Design review of the part built by this model. Coordinates are the model's own, in mm. Face numbers are marked on the shaded views. A direction names the side the tool comes from. Coordinates: 2 decimals unless noted, no trailing zeros. Loops run counter-clockwise (first coordinate to the right, second up) from the corner with the lowest first, then second, coordinate; pieces in that order, holes last. Notation, with made-up numbers: (-17.75, 82.5) - (0.25, 82.5) arc R25 cw to (0.25, 119.5) - close; hole circle Ø11 at (37.25, 43.5). An arc over 180 degrees is marked (long way). Use one line per item in the form item = value. Start each with the question number.
(1) The part is to be moulded in two halves that separate along Z. For the marked faces 3, 4 and 5, say which applies: pulls with the +Z half, pulls with the -Z half, needs draft (parallel to the pull), parting line crosses it, or undercut.
(2) Add section B-B (y = -3.5). State the section outline as (x, z) points.
(3) For L1, parallel to X at y = -4.5, z = -28.5; L2, parallel to X at y = 1.25, z = -12.5; L3, parallel to Z at x = 28, y = -4.25, list the stretches that pass through material, from the lowest coordinate up.
(4) Add section A-A (z = 18.5). State the section outline as (x, y) points, plus the area to 3 significant figures.
(5) Add section C-C (x = 22). State the section outline as (y, z) points.
(6) Add section D-D (z = -33.5). State the section outline as (x, y) points, plus the area to 3 significant figures.
(7) Tool access review of the marked faces 1 and 2: name each direction out of +Z, -Z, +X, -X, +Y, -Y from which nothing blocks a thin tool from reaching the whole face with its end or side.
(8) Clearance check with flat-ended pins moving along their axes: pin 1 Ø5 at (y, z) = (1.5, 20) entering from -X; pin 2 Ø3 at (x, y) = (16, 2) entering from +Z; pin 3 Ø3 at (y, z) = (2.5, -16.5) entering from +X. State where each tip first meets the part, or that it passes through.
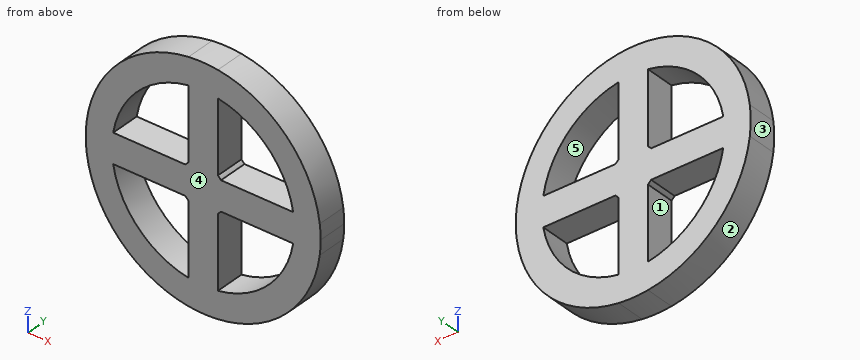
```python
from build123d import *

# Parameters (mm, degrees)
F1_DEPTH = 5


with BuildPart() as f1:
    # F0 (on Front) → F1 (new body, symmetric)
    with BuildSketch(Plane.XZ):
        with BuildLine():
            ThreePointArc((39.68627, -5), (39.92149, -2.504917), (40, 0))
            ThreePointArc((40, 0), (39.92149, 2.504917), (39.68627, 5))
            ThreePointArc((39.68627, 5), (28.284271, 28.284271), (5, 39.68627))
            ThreePointArc((5, 39.68627), (0, 40), (-5, 39.68627))
            ThreePointArc((-5, 39.68627), (-28.284271, 28.284271), (-39.68627, 5))
            ThreePointArc((-39.68627, 5), (-40, 0), (-39.68627, -5))
            ThreePointArc((-39.68627, -5), (-28.284271, -28.284271), (-5, -39.68627))
            ThreePointArc((-5, -39.68627), (0, -40), (5, -39.68627))
            ThreePointArc((5, -39.68627), (28.284271, -28.284271), (39.68627, -5))
        make_face()
        with BuildLine():
            ThreePointArc((-5, -30.641942), (-21.953686, -21.953686), (-30.641942, -5))
            Line((-30.641942, -5), (-6.05909, -5))
            ThreePointArc((-6.05909, -5), (-5.554843, -5.554844), (-5, -6.05909))
            Line((-5, -6.05909), (-5, -30.641942))
        make_face(mode=Mode.SUBTRACT)
        with BuildLine():
            ThreePointArc((5, -6.05909), (5.554843, -5.554843), (6.05909, -5))
            Line((6.05909, -5), (30.641942, -5))
            ThreePointArc((30.641942, -5), (21.953686, -21.953686), (5, -30.641942))
            Line((5, -30.641942), (5, -6.05909))
        make_face(mode=Mode.SUBTRACT)
        with BuildLine():
            ThreePointArc((-30.641942, 5), (-21.953686, 21.953686), (-5, 30.641942))
            Line((-5, 30.641942), (-5, 6.05909))
            ThreePointArc((-5, 6.05909), (-5.554843, 5.554843), (-6.05909, 5))
            Line((-6.05909, 5), (-30.641942, 5))
        make_face(mode=Mode.SUBTRACT)
        with BuildLine():
            Line((30.641942, 5), (6.05909, 5))
            ThreePointArc((6.05909, 5), (5.554843, 5.554843), (5, 6.05909))
            Line((5, 6.05909), (5, 30.641942))
            ThreePointArc((5, 30.641942), (21.953686, 21.953686), (30.641942, 5))
        make_face(mode=Mode.SUBTRACT)
    extrude(amount=F1_DEPTH, both=True)


solid = f1.part
```
Computed values:
q1.face_3 = parting line crosses it
q1.face_4 = needs draft
q1.face_5 = undercut
q2.outline = (-39.69, -5) arc R40 ccw to (-5, -39.69) arc R40 ccw to (5, -39.69) arc R40 ccw to (39.69, -5) arc R40 ccw to (40, 0) arc R40 ccw to (39.69, 5) arc R40 ccw to (5, 39.69) arc R40 ccw to (-5, 39.69) arc R40 ccw to (-39.69, 5) arc R40 ccw to start; hole (-30.64, -5) arc R31.05 ccw to (-5, -30.64) - (-5, -6.06) arc R7.86 cw to (-6.06, -5) - close; hole (-30.64, 5) - (-6.06, 5) arc R7.86 cw to (-5, 6.06) - (-5, 30.64) arc R31.05 ccw to start; hole (5, -30.64) arc R31.05 ccw to (30.64, -5) - (6.06, -5) arc R7.86 cw to (5, -6.06) - close; hole (5, 6.06) arc R7.86 cw to (6.06, 5) - (30.64, 5) arc R31.05 ccw to (5, 30.64) - close
q3.L1 = -28.07 to -12.32, -5 to 5, 12.32 to 28.07
q3.L2 = -38 to -28.42, -5 to 5, 28.42 to 38
q3.L3 = -28.57 to -13.41, -5 to 5, 13.41 to 28.57
q4.outline = (-35.46, -5) - (-24.93, -5) - (-24.93, 5) - (-35.46, 5) - close; (-5, -5) - (5, -5) - (5, 5) - (-5, 5) - close; (24.93, -5) - (35.46, -5) - (35.46, 5) - (24.93, 5) - close
q4.area = 311 mm^2
q5.outline = (-5, -33.41) - (5, -33.41) - (5, -21.91) - (-5, -21.91) - close; (-5, -5) - (5, -5) - (5, 5) - (-5, 5) - close; (-5, 21.91) - (5, 21.91) - (5, 33.41) - (-5, 33.41) - close
q6.outline = (-21.86, -5) - (21.86, -5) - (21.86, 5) - (-21.86, 5) - close
q6.area = 437 mm^2
q7.face_1 = +Y, -Y
q7.face_2 = -Z, -X, +Y, -Y
q8.pin_1 = -35.97
q8.pin_2 = 37.28
q8.pin_3 = 37.08
